Geometry: see drawing. Coordinates: mm, zero at the bounding-box minimum. Give positions to 0.01 mm unless a question says otherwise; leave off trailing zeros. Write each loop counter-clockwise with the first axis right and the second up, starting at its lowest first coordinate (ties: lowest second). Pieces come first, ordered by that corner, then holes. Notation, with made-up numbers: (-8, -11) -> (25, -11) arc R27 ccw to (25, 19) -> close; hole circle Ø5 at (4, 6.5). An arc over 180 degrees is marked (long way). Use CSV: the item, a comma, the result in double quotes. Start each with the question number.
1) Section D-D (z = 18.5). Output: boundary loops of the cut face in (x, y), plus the area to 3 significant figures.
2) Section C-C (x = 6). Output: boundary loops of the cut face in (y, z) (3 decimals), plus the area to 3 significant figures.
3) Contact query for a flat-ended pin moving along its axis: P1, Ø1.5, axis at x = 25, z = 10, coming from the +Y side. Output: stop coordinate, or through.
4) Section B-B (y = 13.5). Output: boundary loops of the cut face in (x, z) (3 decimals), plus the area to 3 significant figures.
5) Material intervals for line 1 (X direction, y = 14.75, z = 10) (3 decimals); line 2 (Z direction, x = 6, y = 9.75) (3 decimals); line 3 (Z direction, x = 1.5, y = 1.25), sorted ascending. Write a range as [from, to].
6) Section A-A (z = 10). Output: boundary loops of the cut face in (x, y) (3 decimals).
7) Draft query along X for the marked faces 1, 2 and 3. Return one class per face: pulls with the +X half, pulls with the -X half, needs draft (parallel to the pull), parting line crosses it, or undercut.
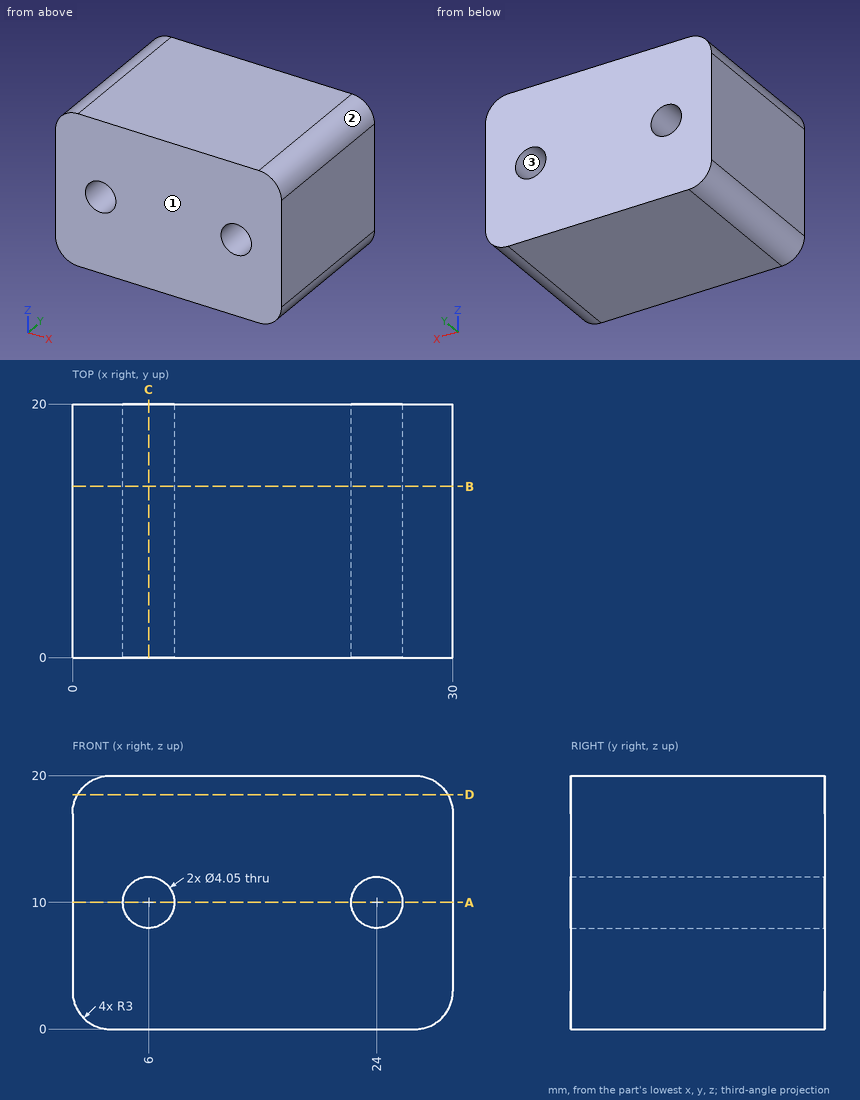
Answers follow:
1,outline,"(0.4, 0) -> (29.6, 0) -> (29.6, 20) -> (0.4, 20) -> close"
1,area,"584 mm^2"
2,outline,"(0, 0) -> (20, 0) -> (20, 7.975) -> (0, 7.975) -> close; (0, 12.025) -> (20, 12.025) -> (20, 20) -> (0, 20) -> close"
2,area,"319 mm^2"
3,P1,"passes through"
4,outline,"(0, 3) arc R3 ccw to (3, 0) -> (27, 0) arc R3 ccw to (30, 3) -> (30, 17) arc R3 ccw to (27, 20) -> (3, 20) arc R3 ccw to (0, 17) -> close; hole circle Ø4.05 at (6, 10); hole circle Ø4.05 at (24, 10)"
4,area,"567 mm^2"
5,line 1,"x = [0, 3.975], [8.025, 21.975], [26.025, 30]"
5,line 2,"z = [0, 7.975], [12.025, 20]"
5,line 3,"z = [0.4, 19.6]"
6,outline,"(0, 0) -> (3.975, 0) -> (3.975, 20) -> (0, 20) -> close; (8.025, 0) -> (21.975, 0) -> (21.975, 20) -> (8.025, 20) -> close; (26.025, 0) -> (30, 0) -> (30, 20) -> (26.025, 20) -> close"
7,face 1,"needs draft"
7,face 2,"pulls with the +X half"
7,face 3,"undercut"
